The drawing under review shows one solid part. Ordinate dimensions are in mm from its lowest x, y, z. A direction names the side the tool comes from. Round coordinates to 2 decimals unless told otherwise and drop trailing zeros. Order: outer loops, then holes, each group sorted by start corner. A loop starts at its lowest first (then second) coordinate and runs counter-clockwise, first axis right, second up. Notation, with made-up numbers: M 44.25,-17 L 53.25,-17 A33 cw 53.25,14 Z; hole C 50,85.25 d6. An arc over 180 degrees is marked long. Answer as a JSON object with one key per item and string values.
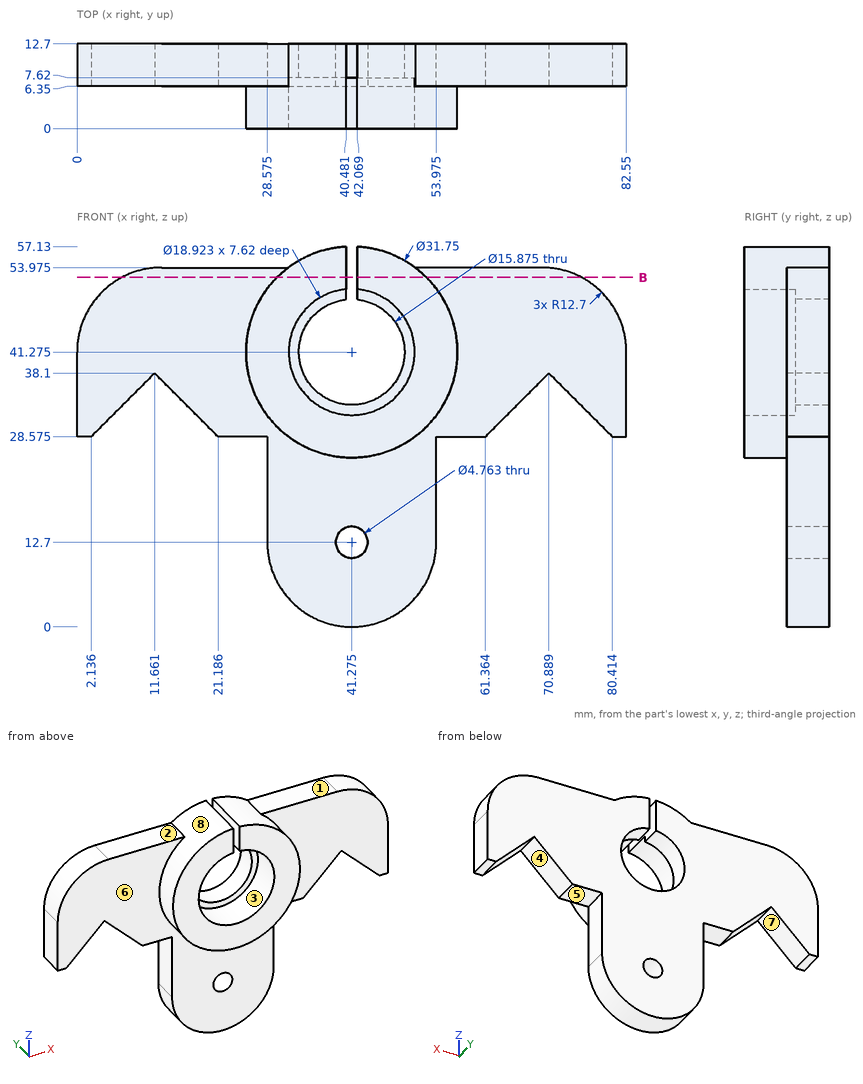
1) For L1, parallel to X at y = 9.5, z = 41.5; L2, parallel to X at y = 8, z = 12.7 (1 decimal); L3, parallel to Y at x = 4, z = 36, list the stretches that pass through material, from the lowest coordinate up.
Geometry check:
{"L1": "x = 0 to 33.34, 49.21 to 82.55", "L2": "x = 28.6 to 38.9, 43.7 to 54", "L3": "y = 6.35 to 12.7"}
2) Mouldability with a two-part tool opening along X and no side actions: class the marked faces 6, 7 and 8 as +X half, -X half, draft (parallel to the pull), parting line (faces both ways), or undercut.
Geometry check:
{"face 6": "draft", "face 7": "undercut", "face 8": "parting line"}
3) Insertion check: P1, Ø3, axis at x = 59, y = 10, coming from the -Z side (1 decimal); P2, Ø2, axis at x = 18, y = 11, coming from the +Z side (1 decimal); P3, Ø5, axis at y = 10, z = 19.5, coming from the -X side (1 decimal); P4, Ø3, axis at y = 3.5, z = 19.5, coming from the -X side. Each pin has a flat end and moves straight along its axis. Give the tip position at first contact, or say it passes through.
Geometry check:
{"P1": "stops at z = 28.6", "P2": "stops at z = 54", "P3": "stops at x = 28.6", "P4": "passes through"}
4) Add section B-B on z = 52.5. State the section outline as (x, y) points, and give its area (3 significant figures).
Geometry check:
{"outline": "M 6.76,6.35 L 30.05,6.35 L 30.05,0 L 40.48,0 L 40.48,12.7 L 6.76,12.7 Z; M 42.07,0 L 52.5,0 L 52.5,6.35 L 75.79,6.35 L 75.79,12.7 L 42.07,12.7 Z", "area": "561 mm²"}
5) Machinability: for the marked faces 1, 2, 3, 4 and 5, which of the approach directions +Z, -Z, +X, -X, +Y, -Y give a long, thin tool a straight path to every point of the face, cutting with its end or side? Answer none if there is none.
Geometry check:
{"face 1": "+Z, +X, +Y, -Y", "face 2": "+Z, -X, +Y, -Y", "face 3": "-Y", "face 4": "-Z, +Y, -Y", "face 5": "-Z, +X, +Y, -Y"}
